Geometry check sheet. Reference: the model listing, model coordinates, mm. Face numbers are marked on the shaded views. A direction names the side the tool comes from. Coordinates: 2 decimals unless noted, no trailing zeros. Write each loop counter-clockwise with the first axis right and the second up, starting at its lowest first coordinate (ties: lowest second). Pieces come first, ordered by that corner, then holes. Notation, with made-up numbers: (-33.5, 12.5) -> (3.5, 12.5) arc R22 ccw to (3.5, 26.5) -> close; hole circle Ø1 at (-32.75, -4). An arc over 180 degrees is marked (long way). Put each result on its own line as item: value. Start each with the question number.
from build123d import *

# Parameters (mm, degrees)
SKETCH1_R           = 11
SKETCH1_R_2         = 1
BOSS_EXTRUDE1_DEPTH = 12
SKETCH2_R           = 3.5
CUT_EXTRUDE1_DEPTH  = 20.646882704
CUT_EXTRUDE2_START  = -8
SKETCH3_R           = 11
SKETCH3_R_2         = 5
CUT_EXTRUDE2_DEPTH  = 8
SKETCH4_W           = 1.5
SKETCH4_H           = 3
CUT_EXTRUDE3_DEPTH  = 4


with BuildPart() as part:
    # Sketch1 → Boss-Extrude1 (new body)
    with BuildSketch(Plane(origin=(0, 0, 0), x_dir=(1, 0, 0), z_dir=(0, 1, 0))):
        with Locations(Location((0, 0, 0), (0, 0, 270))):
            Circle(SKETCH1_R)
        with Locations(Location((0, 8, 0), (0, 0, 270))):
            Circle(SKETCH1_R_2, mode=Mode.SUBTRACT)
        with Locations(Location((5.656854249, 5.656854249, 0), (0, 0, 270))):
            Circle(SKETCH1_R_2, mode=Mode.SUBTRACT)
        with Locations(Location((8, 0, 0), (0, 0, 270))):
            Circle(SKETCH1_R_2, mode=Mode.SUBTRACT)
        with Locations(Location((5.656854249, -5.656854249, 0), (0, 0, 270))):
            Circle(SKETCH1_R_2, mode=Mode.SUBTRACT)
        with Locations(Location((0, -8, 0), (0, 0, 270))):
            Circle(SKETCH1_R_2, mode=Mode.SUBTRACT)
        with Locations(Location((-5.656854249, -5.656854249, 0), (0, 0, 270))):
            Circle(SKETCH1_R_2, mode=Mode.SUBTRACT)
        with Locations(Location((-8, 0, 0), (0, 0, 270))):
            Circle(SKETCH1_R_2, mode=Mode.SUBTRACT)
        with Locations(Location((-5.656854249, 5.656854249, 0), (0, 0, 270))):
            Circle(SKETCH1_R_2, mode=Mode.SUBTRACT)
    extrude(amount=BOSS_EXTRUDE1_DEPTH)

    # Sketch2 → Cut-Extrude1 (cut, through all)
    with BuildSketch(Plane(origin=(0, 12, 0), x_dir=(1, 0, 0), z_dir=(0, 1, 0))):
        with Locations(Location((0, 0, 0), (0, 0, 270))):
            Circle(SKETCH2_R)
    extrude(amount=-CUT_EXTRUDE1_DEPTH, mode=Mode.SUBTRACT)

    # Sketch3 → Cut-Extrude2 (cut)
    with BuildSketch(Plane(origin=(0, 10, 0), x_dir=(1, 0, 0), z_dir=(0, 1, 0)).offset(CUT_EXTRUDE2_START)):
        with Locations(Location((0, 0, 0), (0, 0, 270))):
            Circle(SKETCH3_R)
        with Locations(Location((0, 0, 0), (0, 0, 270))):
            Circle(SKETCH3_R_2, mode=Mode.SUBTRACT)
    extrude(amount=CUT_EXTRUDE2_DEPTH, mode=Mode.SUBTRACT)

    # Sketch4 → Cut-Extrude3 (cut)
    with BuildSketch(Plane(origin=(0, 12, 0), x_dir=(1, 0, 0), z_dir=(0, 1, 0))):
        with Locations((0, 11)):
            Rectangle(SKETCH4_W, SKETCH4_H)
    extrude(amount=-CUT_EXTRUDE3_DEPTH, mode=Mode.SUBTRACT)


solid = part.part
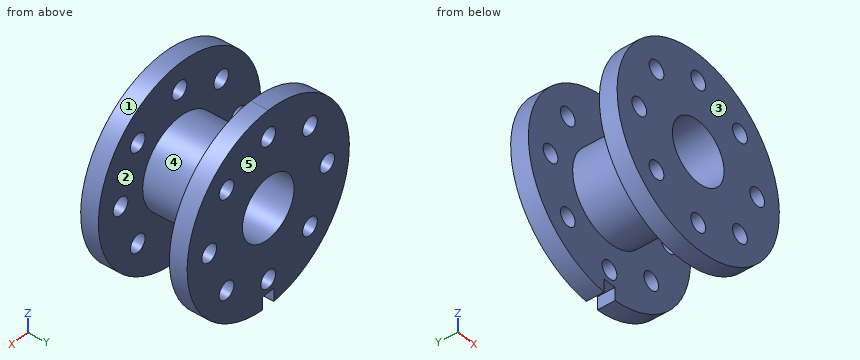
Item 1: Mould release check, pull along Y, two halves, no side actions. Record for the marked faces 3, 4 and 5: released by +Y, released by -Y, zero draft, split by the parting line, or undercut.
Item 2: Go/stop test with flat-tipped pins: P1, Ø3, axis at y = 8, z = -3.5, coming from the +X side; P2, Ø1.2, axis at x = 0.5, y = 11, coming from the -Z side. Record where each tip stops, or that it passes through.
Item 3: Scan lines: line 1 along X through (y, z) = (1.35, 0); line 2 along Y through (x, z) = (8.5, 1.25); line 3 along X through (y, z) = (10.25, 4.75). Record each from-to range of solid material in increasing order. Write a range as [from, to].
Item 4: Section check B-B, the plane z = 8. Enter the section's corners in (x, y), and give its area (3 significant figures).
Item 5: Section check D-D, the plane y = 7. Enter the section's corners in (x, z), and give its area (3 significant figures).
Item 6: Access from +Z, -Z, +X, -X, +Y, -Y to the whole of each face (thin tool, end or side, straight path). Record for the marked faces 1 and 2.
Item 7: Section check C-C, the plane x = -8. Enter the section's corners in (y, z), and give its area (3 significant figures).
Item 8: Section check A-A, the plane x = 1.5. Enter the section's corners in (y, z), and give its area (3 significant figures).
From the geometry:
1. face 3: released by -Y
1. face 4: undercut
1. face 5: released by +Y
2. P1: x = 4.58
2. P2: z = -10.97
3. line 1: [-11, -9], [-7, -3.5], [3.5, 7], [9, 11]
3. line 2: [0, 2], [10, 12]
3. line 3: [-9.92, -6.08], [-5.24, 5.24], [6.08, 9.92]
4. outline: (-7.55, 0) -> (-1, 0) -> (-1, 2) -> (-7.55, 2) -> close; (-7.55, 10) -> (-1, 10) -> (-1, 12) -> (-7.55, 12) -> close; (1, 0) -> (7.55, 0) -> (7.55, 2) -> (1, 2) -> close; (1, 10) -> (7.55, 10) -> (7.55, 12) -> (1, 12) -> close
4. area: 52.4 mm²
5. outline: circle Ø10 at (0, 0); hole circle Ø7 at (0, 0)
5. area: 40.1 mm²
6. face 1: +Y, -Y
6. face 2: none
7. outline: (0, -7.55) -> (2, -7.55) -> (2, -1) -> (0, -1) -> close; (0, 1) -> (2, 1) -> (2, 7.55) -> (0, 7.55) -> close; (10, -7.55) -> (12, -7.55) -> (12, -1) -> (10, -1) -> close; (10, 1) -> (12, 1) -> (12, 7.55) -> (10, 7.55) -> close
7. area: 52.4 mm²
8. outline: (0, -10.9) -> (2, -10.9) -> (2, -4.77) -> (10, -4.77) -> (10, -10.9) -> (12, -10.9) -> (12, -3.16) -> (0, -3.16) -> close; (0, 3.16) -> (12, 3.16) -> (12, 10.9) -> (10, 10.9) -> (10, 4.77) -> (2, 4.77) -> (2, 10.9) -> (0, 10.9) -> close
8. area: 87.6 mm²
